from build123d import *

# Parameters (mm, degrees)
SKETCH1_R              = 45
THAN_CHINH_DEPTH       = 24
SKETCH2_R              = 2.5
VAU_BAT_VIT_DEPTH      = 24
SKETCH3_W              = 14
SKETCH3_H              = 7.5
TAI_RA_DAY_DEPTH       = 24
SKETCH4_R              = 1.25
F_8XM3_MAT_SAU_DEPTH   = 6
F_8XM3_MAT_TRUOC_START = -6
SKETCH5_R              = 1.25
F_8XM3_MAT_TRUOC_DEPTH = 6
SKETCH6_R              = 28.5
ONG_SAU_D57_DEPTH      = 2
SKETCH8_R              = 1.25
F_4XM3_ONG_SAU_DEPTH   = 5
SKETCH9_R              = 30
BAC_D60_DEPTH          = 0.7
SKETCH10_R             = 25
GO_DINH_VI_D50_DEPTH   = 4.1
SKETCH11_R             = 1.25
F_6XM3_DAU_RA_DEPTH    = 5
SKETCH12_R             = 2
F_3XCHOT_D4_DEPTH      = 3.5


with BuildPart() as part:
    # Sketch1 → Than_chinh (new body)
    with BuildSketch(Plane.XY):
        Circle(SKETCH1_R)
    extrude(amount=THAN_CHINH_DEPTH)

    # Sketch2 → Vau_bat_vit (add)
    with BuildSketch(Plane.XY):
        with Locations((42.498458496, 17.603437889)):
            Circle(SKETCH2_R)
        with Locations((17.603437889, 42.498458496)):
            Circle(SKETCH2_R)
        with Locations((-17.603437889, 42.498458496)):
            Circle(SKETCH2_R)
        with Locations((-42.498458496, 17.603437889)):
            Circle(SKETCH2_R)
        with Locations((-42.498458496, -17.603437889)):
            Circle(SKETCH2_R)
        with Locations((-17.603437889, -42.498458496)):
            Circle(SKETCH2_R)
        with Locations((17.603437889, -42.498458496)):
            Circle(SKETCH2_R)
        with Locations((42.498458496, -17.603437889)):
            Circle(SKETCH2_R)
    extrude(amount=VAU_BAT_VIT_DEPTH)

    # Sketch3 → Tai_ra_day (add)
    with BuildSketch(Plane.XY):
        with Locations((0, 44.75)):
            Rectangle(SKETCH3_W, SKETCH3_H)
    extrude(amount=TAI_RA_DAY_DEPTH)

    # Sketch4 → 8xM3_mat_sau (cut)
    with BuildSketch(Plane.XY.offset(24)):
        with Locations((42.498458496, 17.603437889)):
            Circle(SKETCH4_R)
        with Locations((17.603437889, 42.498458496)):
            Circle(SKETCH4_R)
        with Locations((-17.603437889, 42.498458496)):
            Circle(SKETCH4_R)
        with Locations((-42.498458496, 17.603437889)):
            Circle(SKETCH4_R)
        with Locations((-42.498458496, -17.603437889)):
            Circle(SKETCH4_R)
        with Locations((-17.603437889, -42.498458496)):
            Circle(SKETCH4_R)
        with Locations((17.603437889, -42.498458496)):
            Circle(SKETCH4_R)
        with Locations((42.498458496, -17.603437889)):
            Circle(SKETCH4_R)
    extrude(amount=-F_8XM3_MAT_SAU_DEPTH, mode=Mode.SUBTRACT)

    # Sketch5 → 8xM3_mat_truoc (cut)
    with BuildSketch(Plane(origin=(0, 0, 0), x_dir=(-1, 0, 0), z_dir=(0, 0, -1)).offset(F_8XM3_MAT_TRUOC_START)):
        with Locations(Location((-42.498458496, 17.603437889, 0), (0, 0, 180))):
            Circle(SKETCH5_R)
        with Locations(Location((-17.603437889, 42.498458496, 0), (0, 0, 180))):
            Circle(SKETCH5_R)
        with Locations(Location((17.603437889, 42.498458496, 0), (0, 0, 180))):
            Circle(SKETCH5_R)
        with Locations(Location((42.498458496, 17.603437889, 0), (0, 0, 180))):
            Circle(SKETCH5_R)
        with Locations(Location((42.498458496, -17.603437889, 0), (0, 0, 180))):
            Circle(SKETCH5_R)
        with Locations(Location((17.603437889, -42.498458496, 0), (0, 0, 180))):
            Circle(SKETCH5_R)
        with Locations(Location((-17.603437889, -42.498458496, 0), (0, 0, 180))):
            Circle(SKETCH5_R)
        with Locations(Location((-42.498458496, -17.603437889, 0), (0, 0, 180))):
            Circle(SKETCH5_R)
    extrude(amount=F_8XM3_MAT_TRUOC_DEPTH, mode=Mode.SUBTRACT)

    # Sketch6 → Ong_sau_D57 (add)
    with BuildSketch(Plane.XY.offset(24)):
        Circle(SKETCH6_R)
    extrude(amount=ONG_SAU_D57_DEPTH)

    # Sketch8 → 4xM3_ong_sau (cut)
    with BuildSketch(Plane.XY.offset(26)):
        with Locations((18.384776311, 18.384776311)):
            Circle(SKETCH8_R)
        with Locations((-18.384776311, 18.384776311)):
            Circle(SKETCH8_R)
        with Locations((-18.384776311, -18.384776311)):
            Circle(SKETCH8_R)
        with Locations((18.384776311, -18.384776311)):
            Circle(SKETCH8_R)
    extrude(amount=-F_4XM3_ONG_SAU_DEPTH, mode=Mode.SUBTRACT)

    # Sketch9 → Bac_D60 (add)
    with BuildSketch(Plane(origin=(0, 0, 0), x_dir=(-1, 0, 0), z_dir=(0, 0, -1))):
        with Locations(Location((0, 0, 0), (0, 0, 180))):
            Circle(SKETCH9_R)
    extrude(amount=BAC_D60_DEPTH)

    # Sketch10 → Go_dinh_vi_D50 (add)
    with BuildSketch(Plane(origin=(0, 0, 0), x_dir=(-1, 0, 0), z_dir=(0, 0, -1))):
        Circle(SKETCH10_R)
    extrude(amount=GO_DINH_VI_D50_DEPTH)

    # Sketch11 → 6xM3_dau_ra (cut)
    with BuildSketch(Plane(origin=(0, 0, -4.1), x_dir=(-1, 0, 0), z_dir=(0, 0, -1))):
        with Locations((-12.5, 0)):
            Circle(SKETCH11_R)
        with Locations((-6.25, 10.825317547)):
            Circle(SKETCH11_R)
        with Locations((6.25, 10.825317547)):
            Circle(SKETCH11_R)
        with Locations((12.5, 0)):
            Circle(SKETCH11_R)
        with Locations((6.25, -10.825317547)):
            Circle(SKETCH11_R)
        with Locations((-6.25, -10.825317547)):
            Circle(SKETCH11_R)
    extrude(amount=-F_6XM3_DAU_RA_DEPTH, mode=Mode.SUBTRACT)

    # Sketch12 → 3xChot_D4 (add)
    with BuildSketch(Plane(origin=(0, 0, -4.1), x_dir=(-1, 0, 0), z_dir=(0, 0, -1))):
        with Locations((0, 10.2)):
            Circle(SKETCH12_R)
        with Locations((8.833459119, -5.1)):
            Circle(SKETCH12_R)
        with Locations((-8.833459119, -5.1)):
            Circle(SKETCH12_R)
    extrude(amount=F_3XCHOT_D4_DEPTH)


solid = part.part
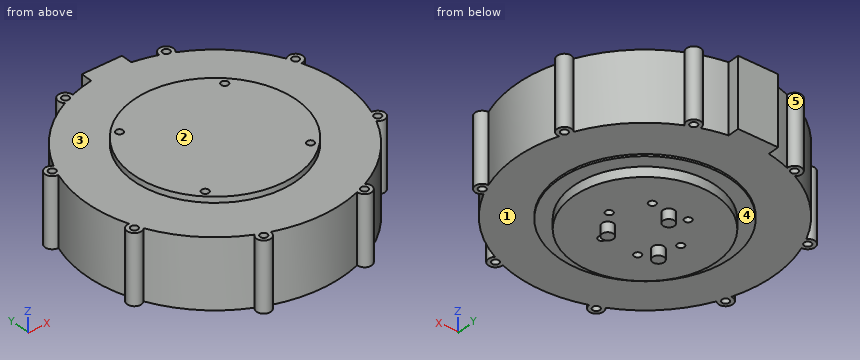
The listing builds one solid part. Answer for the finished solid, in the listing's coordinates (mm). Face numbers are marked on the shaded views. A direction names the side the tool comes from. Give positions to 0.01 mm unless a question says otherwise; leave off trailing zeros. Loops run counter-clockwise (first coordinate to the right, second up) from the corner with the lowest first, then second, coordinate; pieces in that order, holes last.
Item 1: A cutting plane is placed at A-A (y = 0). Give the vertices of the cut face in (x, z).
Derived:
outline: (-45, 0) - (-30, 0) - (-30, -0.7) - (-25, -0.7) - (-25, -4.1) - (-13.75, -4.1) - (-13.75, 0.9) - (-11.25, 0.9) - (-11.25, -4.1) - (11.25, -4.1) - (11.25, 0.9) - (13.75, 0.9) - (13.75, -4.1) - (25, -4.1) - (25, -0.7) - (30, -0.7) - (30, 0) - (45, 0) - (45, 24) - (28.5, 24) - (28.5, 26) - (-28.5, 26) - (-28.5, 24) - (-45, 24) - close
Item 2: A cutting plane is placed at C-C (x = 12.5). Give the vertices of the cut face in (y, z), then the cut area to 3 significant figures.
Derived:
outline: (-43.23, 0) - (-27.27, 0) - (-27.27, -0.7) - (-21.65, -0.7) - (-21.65, -4.1) - (-1.25, -4.1) - (-1.25, 0.9) - (1.25, 0.9) - (1.25, -4.1) - (21.65, -4.1) - (21.65, -0.7) - (27.27, -0.7) - (27.27, 0) - (43.23, 0) - (43.23, 24) - (25.61, 24) - (25.61, 26) - (-25.61, 26) - (-25.61, 24) - (-43.23, 24) - close
area: 2,350 mm2
Item 3: A tool of negligible diameter and unlimited length cuts with its end or side. For the marked faces 1, 2 and 3, from which of +Z, -Z, +X, -X, +Y, -Y can it reach the whole face along a straight path? Write none if from no direction.
Derived:
face 1: -Z
face 2: +Z, +X, -X, +Y, -Y
face 3: +Z
Item 4: A cutting plane is placed at D-D (x = 36). Give the vertices of the cut face in (y, z).
Derived:
outline: (-27, 0) - (27, 0) - (27, 24) - (-27, 24) - close
Item 5: Find the intervals of material crossed by line 1 along Y through (x, z) = (6.25, -2.5); line 2 along Y through (x, z) = (-17, 19.5); line 3 along Z through (x, y) = (19, 26.5), in increasing order.
Derived:
line 1: y = -24.21 to -12.08, -9.58 to 9.58, 12.08 to 24.21
line 2: y = -44.92 to -43.59, -41.4 to 41.4, 43.59 to 44.92
line 3: z = 0 to 24
Item 6: A cutting plane is placed at B-B (x = 0). Give the vertices of the cut face in (y, z).
Derived:
outline: (-45, 0) - (-30, 0) - (-30, -0.7) - (-25, -0.7) - (-25, -4.1) - (8.2, -4.1) - (8.2, -7.6) - (12.2, -7.6) - (12.2, -4.1) - (25, -4.1) - (25, -0.7) - (30, -0.7) - (30, 0) - (48.5, 0) - (48.5, 24) - (28.5, 24) - (28.5, 26) - (-28.5, 26) - (-28.5, 24) - (-45, 24) - close
Item 7: Determine the mould class of the marked faces 4 and 5 for opening direction X: +X half, -X half, draft (parallel to the pull), parting line (faces both ways), or undercut.
Derived:
face 4: draft
face 5: undercut
Item 8: Each of these flat-tipped pins is pushed along its axis until it touches: pin 1 Ø1 at (y, z) = (-19.5, 8) entering from +X; pin 2 Ø3 at (x, y) = (-42.5, 17.6) entering from +Z; pin 3 Ø8 at (x, z) = (-35.5, 10.5) entering from +Y. Where does it stop, or does it pass through?
Derived:
pin 1: stops at x = 44.57
pin 2: stops at z = 24
pin 3: stops at y = 32.14
